from build123d import *

# Parameters (mm, degrees)
SKETCH1_W           = 64
SKETCH1_H           = 86
BOSS_EXTRUDE1_DEPTH = 10
SKETCH2_W           = 64
SKETCH2_H           = 10
BOSS_EXTRUDE2_DEPTH = 40
SKETCH4_R           = 6
SKETCH4_R_2         = 2.25
SKETCH4_R_3         = 3.5
SKETCH4_R_4         = 6.5
CUT_EXTRUDE1_DEPTH  = 11
SKETCH6_R           = 2
SKETCH6_R_2         = 1.25
CUT_EXTRUDE2_DEPTH  = 11
CHAMFER1_SIZE       = 4
FILLET1_R           = 4


with BuildPart() as part:
    # Sketch1 → Boss-Extrude1 (new body)
    with BuildSketch(Plane.XY):
        Rectangle(SKETCH1_W, SKETCH1_H)
    extrude(amount=BOSS_EXTRUDE1_DEPTH)

    # Sketch2 → Boss-Extrude2 (add)
    with BuildSketch(Plane(origin=(0, 0, 0), x_dir=(-1, 0, 0), z_dir=(0, 0, -1))):
        with Locations((0, -38)):
            Rectangle(SKETCH2_W, SKETCH2_H)
    extrude(amount=BOSS_EXTRUDE2_DEPTH)

    # Sketch4 → Cut-Extrude1 (cut, through all)
    with BuildSketch(Plane(origin=(0, 0, 0), x_dir=(-1, 0, 0), z_dir=(0, 0, -1))):
        with Locations((20, 31)):
            Circle(SKETCH4_R)
        with Locations((1, 29)):
            Circle(SKETCH4_R_2)
        with Locations((-20, 31)):
            Circle(SKETCH4_R)
        with Locations((-9, 18)):
            Circle(SKETCH4_R_3)
        with Locations((-23, 18)):
            Circle(SKETCH4_R_3)
        with Locations((18.5, 9)):
            Circle(SKETCH4_R_2)
        with Locations((0, -8)):
            Circle(SKETCH4_R_4)
    extrude(amount=-CUT_EXTRUDE1_DEPTH, mode=Mode.SUBTRACT)

    # Sketch6 → Cut-Extrude2 (cut, through all)
    with BuildSketch(Plane(origin=(0, -33, 0), x_dir=(1, 0, 0), z_dir=(0, 1, 0))):
        with Locations((0, 16.5)):
            Circle(SKETCH6_R)
        with Locations((5.25, 21.75)):
            Circle(SKETCH6_R_2)
        with Locations((5.25, 11.25)):
            Circle(SKETCH6_R_2)
        with Locations((-5.25, 11.25)):
            Circle(SKETCH6_R_2)
        with Locations((-5.25, 21.75)):
            Circle(SKETCH6_R_2)
        with Locations((-9.545941546, 16.5)):
            Circle(SKETCH6_R)
        with Locations((0, 6.954058454)):
            Circle(SKETCH6_R)
        with Locations((9.545941546, 16.5)):
            Circle(SKETCH6_R)
        with Locations((0, 26.045941546)):
            Circle(SKETCH6_R)
    extrude(amount=-CUT_EXTRUDE2_DEPTH, mode=Mode.SUBTRACT)

    # Chamfer1
    chamfer1_edges = [part.edges().sort_by_distance(p)[0] for p in [
        (0, -33, 0),
    ]]
    chamfer(chamfer1_edges, length=CHAMFER1_SIZE)

    # Fillet1
    fillet1_edges = [part.edges().sort_by_distance(p)[0] for p in [
        (0, -43, 10),
    ]]
    fillet(fillet1_edges, radius=FILLET1_R)


solid = part.part
The listing builds one solid part. Answer for the finished solid, in the listing's coordinates (mm). A direction names the side the tool comes from. Coordinates: 2 decimals unless noted, no trailing zeros. Order: outer loops, then holes, each group sorted by start corner. A loop starts at its lowest first (then second) coordinate and runs counter-clockwise, first axis right, second up.
Q1. Which of the six approach directions +Z, -Z, +X, -X, +Y, -Y give full straight-line access (tool end or side, diameter ignored) to faces 5 (the face through (0, -33, -22)), 6 (the face through (-5.52, -37.93, -20.53))?
Q2. Consider line 1 (Z direction, x = 5.25, y = -35.5); line 2 (X direction, y = -35.75, z = -16.5); line 3 (X direction, y = 19, z = 2). Determine where each line is inside the solid, lowest interval first.
Q3. A cutting plane is placed at D-D, the plane y = 18. Write down the section's boundary in (x, z).
Q4. For a pull along Z with two mould halves and no side action, classify faces 1 (the face through (0, -38, -40)), 2 (the face through (0.448, -41.859, 8.797)), 3 (the face through (-0.512, 26.804, 4.93)), 4 (the face through (-0.434, -37.93, -24.094)) as pulls with the +Z half, pulls with the -Z half, needs draft (parallel to the pull), parting line crosses it, or undercut.
Q5. A cutting plane is placed at C-C, the plane z = -16.5. Write down the section's boundary in (x, y), and give its area (3 significant figures).
Q6. Given P1, Ø2.5, axis at x = 0, z = -6.95, coming from the -Y side; P2, Ø11, axis at x = 9, y = 18, coming from the -Z side; P3, Ø5, axis at x = -9.55, z = -16.5, coming from the -Y side; P4, Ø3, axis at x = 16, y = -30.5, coming from the -Z side, each flat-ended and moving along its own axis, determine where each tip first touches the part or whether it passes through.
Q7. A cutting plane is placed at A-A, the plane z = -21.75. Write down the section's boundary in (x, y).
Q8. A cutting plane is placed at B-B, the plane y = 9. Write down the section's boundary in (x, z), and give its area (3 significant figures).
Answers follow:
1. face 5: -Z, +X, -X, +Y
1. face 6: +Y, -Y
2. line 1: z = -40 to -23, -20.5 to -12.5, -10 to 10
2. line 2: x = -32 to -11.55, -7.55 to -2, 2 to 7.55, 11.55 to 32
2. line 3: x = -32 to 5.65, 12.35 to 19.65, 26.35 to 32
3. outline: (-32, 0) - (5.5, 0) - (5.5, 10) - (-32, 10) - close; (12.5, 0) - (19.5, 0) - (19.5, 10) - (12.5, 10) - close; (26.5, 0) - (32, 0) - (32, 10) - (26.5, 10) - close
4. face 1: pulls with the -Z half
4. face 2: pulls with the +Z half
4. face 3: needs draft
4. face 4: undercut
5. outline: (-32, -43) - (-11.55, -43) - (-11.55, -33) - (-32, -33) - close; (-7.55, -43) - (-2, -43) - (-2, -33) - (-7.55, -33) - close; (2, -43) - (7.55, -43) - (7.55, -33) - (2, -33) - close; (11.55, -43) - (32, -43) - (32, -33) - (11.55, -33) - close
5. area: 520 mm2
6. P1: passes through
6. P2: stops at z = 0
6. P3: stops at y = -43
6. P4: stops at z = -3
7. outline: (-32, -43) - (-6.5, -43) - (-6.5, -33) - (-32, -33) - close; (-4, -43) - (4, -43) - (4, -33) - (-4, -33) - close; (6.5, -43) - (32, -43) - (32, -33) - (6.5, -33) - close
8. outline: (-32, 0) - (-20.75, 0) - (-20.75, 10) - (-32, 10) - close; (-16.25, 0) - (32, 0) - (32, 10) - (-16.25, 10) - close
8. area: 595 mm2
